from build123d import *

# Parameters (mm, degrees)
F0_R     = 10.95
F0_R_2   = 11.1
F1_DEPTH = 7
F2_R     = 2
F3_SIZE  = 2


with BuildPart() as f1:
    # F0 (on Top) → F1 (new body)
    with BuildSketch(Plane.XY):
        with BuildLine():
            ThreePointArc((14.915718, -2.351886), (13.104206, 7.502653), (5.522872, 14.05375))
            ThreePointArc((5.522872, 14.05375), (0, 43), (-5.522872, 14.05375))
            ThreePointArc((-5.522872, 14.05375), (-13.104206, 7.502653), (-14.915718, -2.351886))
            ThreePointArc((-14.915718, -2.351886), (-37.174944, -21.462964), (-9.494652, -11.741447))
            ThreePointArc((-9.494652, -11.741447), (0, -15.1), (9.494652, -11.741447))
            ThreePointArc((9.494652, -11.741447), (37.174944, -21.462964), (14.915718, -2.351886))
        make_face()
        with Locations((-24.248711, -14)):
            Circle(F0_R, mode=Mode.SUBTRACT)
        with Locations((24.248711, -14)):
            Circle(F0_R, mode=Mode.SUBTRACT)
        Circle(F0_R_2, mode=Mode.SUBTRACT)
        with Locations((0, 28)):
            Circle(F0_R, mode=Mode.SUBTRACT)
    extrude(amount=F1_DEPTH)

    # F2
    f2_edges = [f1.edges().sort_by_distance(p)[0] for p in [
        (-9.494652, -11.741447, 3.5),
        (9.494652, -11.741447, 3.5),
        (14.915718, -2.351886, 3.5),
        (5.522872, 14.05375, 3.5),
        (-5.522872, 14.05375, 3.5),
        (-14.915718, -2.351886, 3.5),
    ]]
    fillet(f2_edges, radius=F2_R)

    # F3
    f3_edges = [f1.edges().sort_by_distance(p)[0] for p in [
        (37.174944, -21.462964, 0),
        (37.174944, -21.462964, 7),
    ]]
    chamfer(f3_edges, length=F3_SIZE)


solid = f1.part
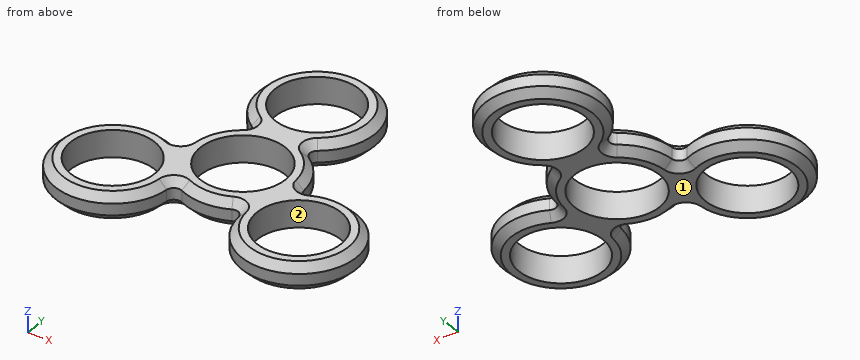
Part model, mm, in its own coordinate system. Face numbers are marked on the shaded views. Coordinates: 2 decimals unless noted, no trailing zeros. Order: outer loops, then holes, each group sorted by start corner. A loop starts at its lowest first (then second) coordinate and runs counter-clockwise, first axis right, second up. Notation, with made-up numbers: M 41,77.25 L 95,77.25 A25 cw 95,101.25 Z; hole C 23,-7 d2. An arc over 180 degrees is marked long. Use a Markdown table: item, result.
(1) Flat gauge pins, fed straight in: pin 1 (8 mm diameter, centred on x = -16.5, y = 26, fed in from -Z); pin 2 (1 mm diameter, centred on x = 18.5, z = 5.5, fed in from +Y); pin 3 (19.5 mm diameter, centred on x = 0, y = 28, fed in from +Z). Where does each tip first touch, or does it go through?
A:
| item | result |
|---|---|
| pin 1 | stops at z = 0 |
| pin 2 | stops at y = -0.19 |
| pin 3 | passes through |
(2) Probe L1, parallel to Y at x = -0.5, z = 2.25; L2, parallel to Y at x = -6, z = 4.5; L3, parallel to Y at x = 28, z = 1.5. List the from-to ranges inside material, lowest first.
A:
| item | result |
|---|---|
| L1 | y = -15.09 to -11.09, 11.09 to 17.06, 38.94 to 42.99 |
| L2 | y = -13.86 to -9.34, 9.34 to 18.84, 37.16 to 41.75 |
| L3 | y = -27.93 to -24.29, -3.71 to -0.07 |
(3) Pull direction X, two halves, no side cores. Call the marked faces 1 and 2: released by +X, released by -X, zero draft, split by the parting line, or undercut.
A:
| item | result |
|---|---|
| face 1 | zero draft |
| face 2 | undercut |
(4) Cut at B-B on y = 28. Write the cut outline in (x, z).
A:
| item | result |
|---|---|
| outline | M -15,2 L -13,0 L -10.95,0 L -10.95,7 L -13,7 L -15,5 Z; M 10.95,0 L 13,0 L 15,2 L 15,5 L 13,7 L 10.95,7 Z |
(5) Cut at A-A on x = 0. Write the cut outline in (y, z), then the cut area to 3 significant figures.
A:
| item | result |
|---|---|
| outline | M -15.1,2 L -13.1,0 L -11.1,0 L -11.1,7 L -13.1,7 L -15.1,5 Z; M 11.1,0 L 17.05,0 L 17.05,7 L 11.1,7 Z; M 38.95,0 L 41,0 L 43,2 L 43,5 L 41,7 L 38.95,7 Z |
| area | 90.0 mm^2 |
(6) Cut at C-C on z = 3.5. State how many separate pieces and enclosed holes the cut face has, then the cut area to 3 significant figures.
A:
| item | result |
|---|---|
| separate pieces | 1 |
| enclosed holes | 4 |
| area | 1,280 mm^2 |
